Verification items for the finished model (mm, model axes). Round coordinates to 2 decimals unless told otherwise and drop trailing zeros. Write each loop counter-clockwise with the first axis right and the second up, starting at its lowest first coordinate (ties: lowest second). Pieces come first, ordered by that corner, then holes. Notation, with made-up numbers: M 85,-33 L 137,-33 A22 cw 137,3 Z; hole C 51.25,60.5 d8. An arc over 180 degrees is marked long. One line per item, written item: value. Start each with the question number.
from build123d import *

# Parameters (mm, degrees)
F0_R          = 10
F1_DEPTH      = 25
F2_DEPTH      = 50
F3_SIZE       = 2
F5_DEPTH      = 25
F5_DEPTH_BACK = 59.7565770149


# Not quite as in the source:
# - the program builds the solid bodies; features that only make, move or delete a surface that nothing else refers to are left out


with BuildPart() as f1:
    # F0 (on Front) → F1 (new body)
    with BuildSketch(Plane.XZ):
        with BuildLine():
            ThreePointArc((2.0833333333, -24.9130432148), (18.3995018048, -16.9250800097), (25, 0))
            ThreePointArc((25, 0), (18.3995018048, 16.9250800097), (2.0833333333, 24.9130432148))
            ThreePointArc((2.0833333333, 24.9130432148), (-25, 0), (2.0833333333, -24.9130432148))
        make_face()
        Circle(F0_R, mode=Mode.SUBTRACT)
        with BuildLine():
            ThreePointArc((2.0833333333, 24.9130432148), (18.3995018048, 16.9250800097), (25, 0))
            ThreePointArc((25, 0), (18.3995018048, -16.9250800097), (2.0833333333, -24.9130432148))
            Line((2.0833333333, -24.9130432148), (91.4583333333, -17.4391302504))
            ThreePointArc((91.4583333333, -17.4391302504), (72.5, 0), (91.4583333333, 17.4391302504))
            Line((91.4583333333, 17.4391302504), (2.0833333333, 24.9130432148))
        make_face()
        with BuildLine():
            ThreePointArc((107.5, 0), (102.8796512634, 11.8475560068), (91.4583333333, 17.4391302504))
            ThreePointArc((91.4583333333, 17.4391302504), (72.5, 0), (91.4583333333, -17.4391302504))
            ThreePointArc((91.4583333333, -17.4391302504), (102.8796512634, -11.8475560068), (107.5, 0))
        make_face()
        with Locations((90, 0)):
            Circle(F0_R, mode=Mode.SUBTRACT)
    extrude(amount=F1_DEPTH)

    # F0 (on Front) → F2 (join)
    with BuildSketch(Plane.XZ):
        with BuildLine():
            ThreePointArc((2.0833333333, -24.9130432148), (18.3995018048, -16.9250800097), (25, 0))
            ThreePointArc((25, 0), (18.3995018048, 16.9250800097), (2.0833333333, 24.9130432148))
            ThreePointArc((2.0833333333, 24.9130432148), (-25, 0), (2.0833333333, -24.9130432148))
        make_face()
        Circle(F0_R, mode=Mode.SUBTRACT)
    extrude(amount=F2_DEPTH)

    # F3
    f3_edges = [f1.edges().sort_by_distance(p)[0] for p in [
        (-2.083333, -50, 24.913043),
        (-10, -50, 0),
        (80, -25, 0),
    ]]
    chamfer(f3_edges, length=F3_SIZE)

    # F0 (on Front) → F5 (join, two sides)
    with BuildSketch(Plane.XZ) as f5_sk:
        with BuildLine():
            ThreePointArc((2.0833333333, -24.9130432148), (18.3995018048, -16.9250800097), (25, 0))
            ThreePointArc((25, 0), (18.3995018048, 16.9250800097), (2.0833333333, 24.9130432148))
            ThreePointArc((2.0833333333, 24.9130432148), (-25, 0), (2.0833333333, -24.9130432148))
        make_face()
        Circle(F0_R, mode=Mode.SUBTRACT)
        with BuildLine():
            ThreePointArc((2.0833333333, 24.9130432148), (18.3995018048, 16.9250800097), (25, 0))
            ThreePointArc((25, 0), (18.3995018048, -16.9250800097), (2.0833333333, -24.9130432148))
            Line((2.0833333333, -24.9130432148), (91.4583333333, -17.4391302504))
            ThreePointArc((91.4583333333, -17.4391302504), (72.5, 0), (91.4583333333, 17.4391302504))
            Line((91.4583333333, 17.4391302504), (2.0833333333, 24.9130432148))
        make_face()
        with BuildLine():
            ThreePointArc((107.5, 0), (102.8796512634, 11.8475560068), (91.4583333333, 17.4391302504))
            ThreePointArc((91.4583333333, 17.4391302504), (72.5, 0), (91.4583333333, -17.4391302504))
            ThreePointArc((91.4583333333, -17.4391302504), (102.8796512634, -11.8475560068), (107.5, 0))
        make_face()
        with Locations((90, 0)):
            Circle(F0_R, mode=Mode.SUBTRACT)
    extrude(amount=F5_DEPTH)
    extrude(f5_sk.sketch, amount=-F5_DEPTH_BACK)


solid = f1.part
1) Mould release check, pull along X, two halves, no side actions. Record for faces 1 (the flat face through (40, 59.757, 0)), 2 (the conical face through (-2.195, -48.125, -9.884)): pulls with the +X half, pulls with the -X half, needs draft (parallel to the pull), parting line crosses it, or undercut.
2) Cross-section at B-B (y = 35). Record the boundary of the cut face in (x, z).
3) Gauge pin test, flat ends, axial feed: pin 1 Ø23 at (x, z) = (90, 0) entering from -Y; pin 2 Ø4 at (y, z) = (6.5, 17.5) entering from -X; pin 3 Ø3 at (y, z) = (-28, 9) entering from -X. Record the tip position at first contact, or that the pin passes through.
4) Cross-section at D-D (x = 90). Record the boundary of the cut face in (y, z).
5) Thickness scan on line 1 (Z direction, x = 0, y = -25.5); line 2 (X direction, y = 47, z = -2); line 3 (Y direction, x = 43, z = -2.5). Record the ranges inside material, lowest first.
6) Cross-section at A-A (x = 0). Record the boundary of the cut face in (y, z), then the cut area to 3 significant figures.
7) Cross-section at C-C (y = -30). Record the boundary of the cut face in (x, z), then the cut area to 3 significant figures.
Results below:
1. face 1: needs draft
1. face 2: undercut
2. outline: M 2.08,-24.91 L 91.46,-17.44 A17.5 ccw 91.46,17.44 L 2.08,24.91 A25 ccw long Z; hole C 0,0 d20; hole C 90,0 d20
3. pin 1: stops at y = -25
3. pin 2: stops at x = -19.62
3. pin 3: stops at x = -23.85
4. outline: M -25,-17.56 L 59.76,-17.56 L 59.76,-10 L -25,-10 Z; M -25,10 L 59.76,10 L 59.76,17.56 L -25,17.56 Z
5. line 1: z = -25 to -10, 10 to 25
5. line 2: x = -24.92 to -9.8, 9.8 to 80.2, 99.8 to 107.39
5. line 3: y = -25 to 59.76
6. outline: M -50,-23 L -48,-25 L 59.76,-25 L 59.76,-10 L -48,-10 L -50,-12 Z; M -50,12 L -48,10 L 59.76,10 L 59.76,25 L -48,25 L -50,23 Z
6. area: 3,280 mm²
7. outline: C 0,0 d50; hole C 0,0 d20
7. area: 1,650 mm²
